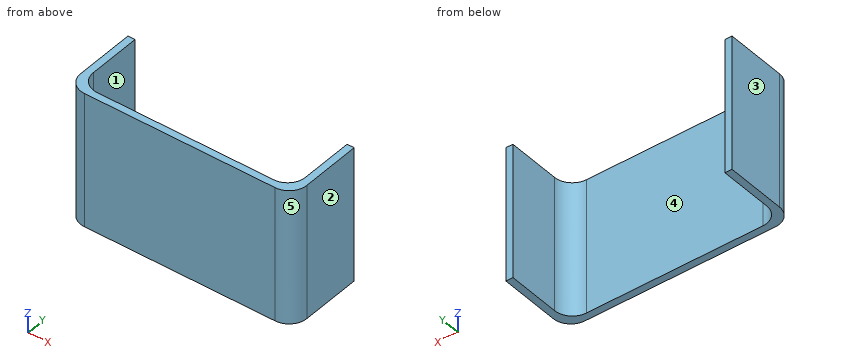
```python
from build123d import *

# Parameters (mm, degrees)
F1_DEPTH = 38


with BuildPart() as f1:
    # F0 (on Top) → F1 (new body)
    with BuildSketch(Plane.XY):
        with BuildLine():
            Line((25, 0), (0, 0))
            Line((0, 0), (-25, 0))
            ThreePointArc((-25, 0), (-28.535534, 1.464466), (-30, 5))
            Line((-30, 5), (-30, 20))
            Line((-30, 20), (-32, 20))
            Line((-32, 20), (-32, 3))
            ThreePointArc((-32, 3), (-30.535534, -0.535534), (-27, -2))
            Line((-27, -2), (0, -2))
            Line((0, -2), (27, -2))
            ThreePointArc((27, -2), (30.535534, -0.535534), (32, 3))
            Line((32, 3), (32, 20))
            Line((32, 20), (30, 20))
            Line((30, 20), (30, 5))
            ThreePointArc((30, 5), (28.535534, 1.464466), (25, 0))
        make_face()
    extrude(amount=F1_DEPTH)


solid = f1.part
```
The model under review builds one solid part; all positions refer to its coordinate system, in mm. Face numbers are marked on the shaded views. A direction names the side the tool comes from. Round coordinates to 2 decimals unless told otherwise and drop trailing zeros. Loops run counter-clockwise (first coordinate to the right, second up) from the corner with the lowest first, then second, coordinate; pieces in that order, holes last. Notation, with made-up numbers: M -36.75,-11 L -16.75,-11 A30 cw -16.75,13 Z; hole C 35,-26.5 d5. An arc over 180 degrees is marked long. Answer as a JSON object with one key per item and string values.
(1) Take a section at A-A on y = 10.75. Give the boundary of the cut face in (x, z).
Resolved:
{"outline": "M -32,0 L -30,0 L -30,38 L -32,38 Z; M 30,0 L 32,0 L 32,38 L 30,38 Z"}
(2) Tool access review of the marked faces 4 and 5: name each direction out of +Z, -Z, +X, -X, +Y, -Y from which nothing blocks a thin tool from reaching the whole face with its end or side.
Resolved:
{"face 4": "+Z, -Z, +Y", "face 5": "+Z, -Z, +X, -Y"}
(3) Take a section at C-C on y = 1.25. Give the boundary of the cut face in (x, z), and give its area (3 significant figures).
Resolved:
{"outline": "M -31.68,0 L -28.31,0 L -28.31,38 L -31.68,38 Z; M 28.31,0 L 31.68,0 L 31.68,38 L 28.31,38 Z", "area": "257 mm²"}
(4) To check wall thickness, follow line 1 along X through (y, z) = (4.75, 7); line 2 along Y through (x, z) = (7, 5); line 3 along Y through (x, z) = (28.5, 18). State the ranges of each line that lie inside material, in increasing order.
Resolved:
{"line 1": "-32 to -29.99, 29.99 to 32", "line 2": "-2 to 0", "line 3": "-1.77 to 1.43"}
(5) Clearance check with flat-ended pins moving along their axes: P1, Ø4, axis at x = -1, z = 7.5, coming from the +Y side; P2, Ø1.5, axis at y = 1, z = 29, coming from the +X side; P3, Ø10, axis at x = -5.5, y = 4, coming from the +Z side. State where each tip first meets the part, or that it passes through.
Resolved:
{"P1": "y = 0", "P2": "x = 31.84", "P3": "z = 38"}
(6) Draft analysis for pull direction X (two halves, no side actions). For the marked faces 1, 2 and 3, state which applies: released by +X, released by -X, zero draft, split by the parting line, or undercut.
Resolved:
{"face 1": "undercut", "face 2": "released by +X", "face 3": "released by -X"}
(7) Take a section at D-D on x = 20.5. Give the boundary of the cut face in (y, z).
Resolved:
{"outline": "M -2,0 L 0,0 L 0,38 L -2,38 Z"}
(8) Take a section at B-B on z = 25.5. Give the boundary of the cut face in (x, y).
Resolved:
{"outline": "M -32,3 A5 ccw -27,-2 L 27,-2 A5 ccw 32,3 L 32,20 L 30,20 L 30,5 A5 cw 25,0 L -25,0 A5 cw -30,5 L -30,20 L -32,20 Z"}
